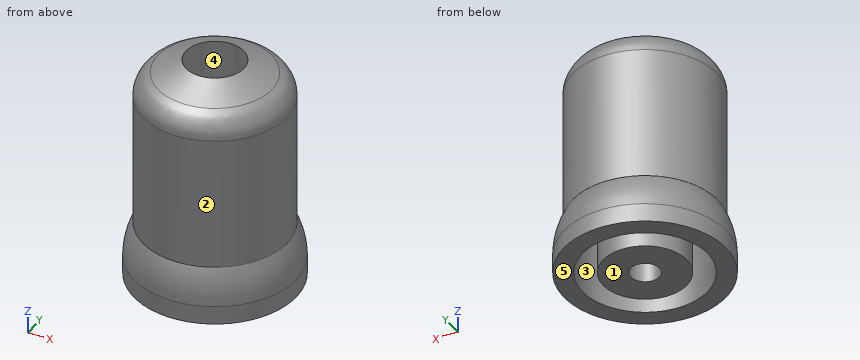
```python
from build123d import *

# Parameters (mm, degrees)
F2_R     = 2.7
F3_DEPTH = 44.201
F4_R     = 11.6
F4_R_2   = 7.75
F5_DEPTH = 38.2
F6_R     = 5
F8_R     = 5.35
F9_DEPTH = 34.1


# Not quite as in the source:
# - a fillet or chamfer that OpenCascade refuses, or shapes differently, is made with other operations: its cross-section is extruded or revolved along the edge and cut away or added


with BuildPart() as f1:
    # F0 (on Front) → F1 (revolve)
    with BuildSketch(Plane.XZ):
        Polygon((0, -25.2708706191), (0, 18.9291293809), (-13.35, 12.5291293809), (-13.35, -15.2708706191), (-15, -15.2708706191), (-15, -25.2708706191), align=None)
    revolve(axis=Axis((0, 0, -3.1708706191), (0, 0, -1)))

    # F2 (on face) → F3 (cut, through all)
    with BuildSketch(Plane(origin=(0, 0, -25.2708706191), x_dir=(1, 0, 0), z_dir=(0, 0, -1))):
        Circle(F2_R)
    extrude(amount=-F3_DEPTH, mode=Mode.SUBTRACT)

    # F4 (on face) → F5 (cut)
    with BuildSketch(Plane(origin=(0, 0, -25.2708706191), x_dir=(1, 0, 0), z_dir=(0, 0, -1))):
        Circle(F4_R)
        Circle(F4_R_2, mode=Mode.SUBTRACT)
    extrude(amount=-F5_DEPTH, mode=Mode.SUBTRACT)

    # F6
    f6_edges = [f1.edges().sort_by_distance(p)[0] for p in [
        (13.35, 0, 12.529129),
    ]]
    fillet(f6_edges, radius=F6_R)

    # F8 (on offset) → F9 (cut)
    with BuildSketch(Plane.XY.offset(17.8)):
        Circle(F8_R)
    extrude(amount=-F9_DEPTH, mode=Mode.SUBTRACT)

    # F10: fillet of radius 14 on 1 edges, made by hand

    # F10_s1 → F10_t2 (revolve, cut)
    with BuildSketch(Plane.XZ):
        with BuildLine():
            ThreePointArc((-13.35, -15.2708706191), (-14.5812370571, -18.4660885634), (-15, -21.864617657))
            Line((-15, -21.864617657), (-15, -15.2708706191))
            Line((-15, -15.2708706191), (-13.35, -15.2708706191))
        make_face()
    revolve(axis=Axis((0, 0, -15.2708706191), (0, 0, -1)), mode=Mode.SUBTRACT)


solid = f1.part
```
The listing builds one solid part. Answer for the finished solid, in the listing's coordinates (mm). Face numbers are marked on the shaded views. A direction names the side the tool comes from. Round coordinates to 2 decimals unless told otherwise and drop trailing zeros. Loops run counter-clockwise (first coordinate to the right, second up) from the corner with the lowest first, then second, coordinate; pieces in that order, holes last.
Q1. Which of the six approach directions +Z, -Z, +X, -X, +Y, -Y give full straight-line access (tool end or side, diameter ignored) to the marked faces 4 and 5?
Q2. Section A-A, the plane z = 6 is taken. Determine the outline of the cut face in (x, y), then the cut area to 3 significant figures.
Q3. Find the intervals of material crossed by line 1 (Y direction, x = 0, z = -13); line 2 (Y direction, x = 0, z = -23), in increasing order.
Q4. For a pull along Y with two mould halves and no side action, classify the marked faces 1, 2 and 3 as released by +Y, released by -Y, zero draft, split by the parting line, or undercut.
Q5. Given pin 1 Ø1.5 at (y, z) = (4, 2) entering from +X; pin 2 Ø12 at (x, y) = (-2.5, 1) entering from +Z; pin 3 Ø8 at (x, z) = (-4.5, 8) entering from +Y; pin 4 Ø6.5 at (x, y) = (0, 0) entering from +Z, each flat-ended and moving along its own axis, determine where each tip first touches the part or whether it passes through.
Q6. Section B-B, the plane z = -17.5 is taken. Count the separate pieces of the cut face and the enclosed holes in it, then the cut area to 3 significant figures.
Completed:
1. face 4: +Z
1. face 5: -Z, +X, -X, +Y, -Y
2. outline: circle Ø26.7 at (0, 0); circle Ø15.5 at (0, 0); hole circle Ø23.2 at (0, 0); hole circle Ø10.7 at (0, 0)
2. area: 236 mm2
3. line 1: y = -13.35 to -11.6, -7.75 to -5.35, 5.35 to 7.75, 11.6 to 13.35
3. line 2: y = -15 to -11.6, -7.75 to -2.7, 2.7 to 7.75, 11.6 to 15
4. face 1: zero draft
4. face 2: split by the parting line
4. face 3: undercut
5. pin 1: stops at x = 12.95
5. pin 2: stops at z = 16.36
5. pin 3: stops at y = 13.34
5. pin 4: stops at z = -16.3
6. separate pieces: 2
6. enclosed holes: 2
6. area: 386 mm2
